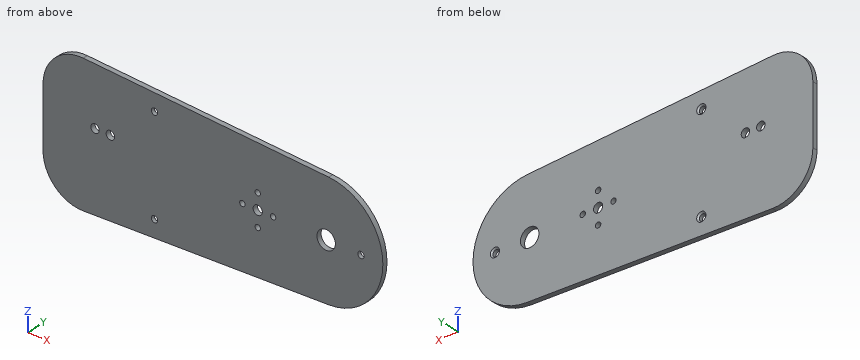
Autodesk Inventor part; units mm, degrees
ref_plane "YZ Plane" through (0, 0, 0) normal (1, 0, 0) x (0, 1, 0)
ref_plane "XZ Plane" through (0, 0, 0) normal (0, 1, 0) x (-1, 0, 0)
ref_plane "XY Plane" through (0, 0, 0) normal (0, 0, 1) x (1, 0, 0)
sketch "Sketch1" plane through (0, 0, 0) normal (0, 1, 0) x (-1, 0, 0)
  arc A0 (-1.6679, 36.7922) -> (-1.6679, -36.7922) centre (0, 0) ccw
  arc A1 (157.8679, -44.0244) -> (184, -19.05) centre (159, -19.05) ccw
  arc A2 (184, 19.05) -> (157.8679, 44.0244) centre (159, 19.05) ccw
  line L0 (157.8679, -44.0244) -> (-1.6679, -36.7922)
  line L1 (157.8679, 44.0244) -> (-1.6679, 36.7922)
  line L2 (184, -19.05) -> (184, 19.05)
  line L3 (0, 0) -> (1115.1702, 0)
  dimension "d0" = 50
  dimension "d1" = 159
  dimension "d2" = 38.1
  dimension "d3" = 36.83
extrude "Main" add sketch "Sketch1" along normal blind 3.175
sketch "Sketch2" plane through (0, 3.175, 0) normal (0, 1, 0) x (1, 0, 0)
  circle A0 centre (0, 0) radius 6
  circle A1 centre (-44.4754, 0) radius 3
  arc A2 (-184, -19.05) -> (-157.8679, -44.0244) centre (-159, -19.05) ccw
  arc A3 (-157.8679, 44.0244) -> (-184, 19.05) centre (-159, 19.05) ccw
  line L0 (0, 0) -> (-245.2379, 0)
  dimension "d6" = 6
  dimension "d40" = 12
  dimension "d41" = 44.4754
extrude "Axis Holes" cut sketch "Sketch2" against normal through all
sketch "Sketch5" plane through (0, 3.175, 0) normal (0, 1, 0) x (1, 0, 0)
  line L0 (-133.2, -6.35) -> (-133.2, 29.1375) construction
  line L1 (-184, 19.05) -> (-184, -19.05) construction
  circle A0 centre (-140.2, -6.35) radius 2.75
  circle A1 centre (-150.2, -6.35) radius 2.75
  point P0 (0, 0)
  dimension "d43" = 50.8
  dimension "d44" = 7
  dimension "d45" = 10
  dimension "d46" = 5.5
extrude "Extrusion6" cut sketch "Sketch5" against normal through all
sketch "Sketch7" plane through (0, 3.175, 0) normal (0, 1, 0) x (1, 0, 0)
  circle A0 centre (-44.4754, 0) radius 3 construction
  circle A1 centre (-44.4754, 0) radius 10 construction
  circle A2 centre (-44.4754, 10) radius 1.75
  circle A3 centre (-54.4754, 0) radius 1.75
  circle A4 centre (-44.4754, -10) radius 1.75
  circle A5 centre (-34.4754, 0) radius 1.75
  point P0 (0, 0)
  dimension "d63" = 20
  dimension "d58" = 3.5
  dimension "d61" = 360
extrude "Extrusion8" cut sketch "Sketch7" against normal blind 10
sketch "Sketch9" plane through (0, 3.175, 0) normal (0, 1, 0) x (1, 0, 0)
  circle A0 centre (-44.4754, 0) radius 3
  point P0 (0, 0)
  point P1 (-12.3688, -17.5481)
  point P2 (-111.5344, -31)
  point P3 (-111.5344, 31)
  point P4 (22.5836, 0)
  dimension "d73" = 67.059
  dimension "d74" = 67.059
  dimension "d75" = 31
  dimension "d76" = 31
hole "Hole1" at (-111.5344, 3.175, 31) at (-111.5344, 3.175, -31) at (22.5836, 3.175, 0) direction (0, -1, 0) diameter 4.134 end through all countersink diameter 6 countersink angle 90
properties part number "Wrist Side Brase" material "Aluminum 6061"
Source: CAD feature listing. Evaluate the final solid. Frame: model axes, mm. Give positions to 0.01 mm unless a question says otherwise; leave off trailing zeros. Loops run counter-clockwise (first coordinate to the right, second up) from the corner with the lowest first, then second, coordinate; pieces in that order, holes last. Notation, with made-up numbers: (9.5, 31.25) -> (64.5, 31.25) arc R12 cw to (64.5, 46.25) -> close; hole circle Ø1 at (23, -13). An arc over 180 degrees is marked (long way). Use a Markdown table: item, result. Add a question column.
1) Section query B-B, the plane z = 31. Return the cut outline in (x, y) (3 decimals).
2) Section query A-A, the plane x = -150.2. Return the cut outline in (y, z) (3 decimals), then the cut area to 3 significant figures.
3) Section query C-C, the plane y = 1.1. Count the separate pieces of the cut face and the enclosed holes in it, then the cut area to 3 significant figures.
4) Section query D-D, the plane x = -119. Return the cut outline in (y, z) (3 decimals).
5) Line query: line 1 along X through (y, z) = (1, 6.35); line 2 along X through (y, z) = (0.4, 8); line 3 along X through (y, z) = (1.3, 32). Output: solid intervals per line, ascending. Write a range as [from, to].
6) First-contact query: pin 1 (4 mm diameter, centred on x = -34.48, z = 0, fed in from -Y); pin 2 (1 mm diameter, centred on y = 2, z = -24.5, fed in from -X). Flat tips, straight axial feed; report the tip coordinate or a pass-through.
Numbers:
| question | item | result |
|---|---|---|
| 1 | outline | (-180.959, 0) -> (-113.601, 0) -> (-113.601, 2.242) -> (-114.534, 3.175) -> (-180.959, 3.175) -> close; (-109.467, 0) -> (19.886, 0) -> (19.886, 3.175) -> (-108.534, 3.175) -> (-109.467, 2.242) -> close |
| 2 | outline | (0, -43.677) -> (3.175, -43.677) -> (3.175, 3.6) -> (0, 3.6) -> close; (0, 9.1) -> (3.175, 9.1) -> (3.175, 43.677) -> (0, 43.677) -> close |
| 2 | area | 260 mm2 |
| 3 | separate pieces | 1 |
| 3 | enclosed holes | 11 |
| 3 | area | 16,700 mm2 |
| 4 | outline | (0, -42.262) -> (3.175, -42.262) -> (3.175, 42.262) -> (0, 42.262) -> close |
| 5 | line 1 | x = [-184, -152.95], [-147.45, -142.95], [-137.45, 36.28] |
| 5 | line 2 | x = [-184, -152.4], [-148, -142.4], [-138, 35.95] |
| 5 | line 3 | x = [-180.38, -113.34], [-109.73, 18.23] |
| 6 | pin 1 | stops at y = 0 |
| 6 | pin 2 | stops at x = -183.51 |
